Design review of the part built by this model. Coordinates are the model's own, in mm. Face numbers are marked on the shaded views. Give positions to 0.01 mm unless a question says otherwise; leave off trailing zeros. Write each loop counter-clockwise with the first axis right and the second up, starting at its lowest first coordinate (ties: lowest second). Pieces come first, ordered by that corner, then holes. Notation, with made-up numbers: (65, -30) -> (114, -30) arc R30 cw to (114, 0) -> close; hole circle Ø3 at (46, -4). An arc over 180 degrees is marked (long way). Answer as a JSON object with one key per item and string values.
Autodesk Fusion 360 part; units mm, degrees
sketch "Sketch1" plane through (0, 0, 0) normal (0, 0, 1) x (1, 0, 0)
  line L0 (10, -60) -> (-10, -60)
  line L1 (-10, -60) -> (-10, 60)
  line L2 (-10, 60) -> (10, 60)
  line L3 (10, 60) -> (10, -60)
  line L4 (10, -60) -> (-10, 60) construction
  line L5 (-10, -60) -> (10, 60) construction
  dimension "d1" = 20
  dimension "d2" = 120
extrude "Extrude1" add sketch "Sketch1" along normal blind 12
sketch "Sketch2" plane through (0, 0, 12) normal (0, 0, 1) x (-1, 0, 0)
  line L0 (-10, -60) -> (10, -60)
  line L1 (10, -60) -> (10, 60)
  line L2 (10, 60) -> (-10, 60)
  line L3 (-10, 60) -> (-10, -60)
  circle A0 centre (0, -50) radius 2
  circle A1 centre (0, 50) radius 2
extrude "Extrude2" cut sketch "Sketch2" against normal blind 12 contours A0
sketch "Sketch3" plane through (0, 0, 12) normal (0, 0, 1) x (-1, 0, 0)
  circle A0 centre (0, -50) radius 2
  line L0 (-10, -60) -> (10, -60)
  line L1 (10, -60) -> (10, 60)
  line L2 (10, 60) -> (-10, 60)
  line L3 (-10, 60) -> (-10, -60)
  circle A1 centre (0, 50) radius 2
  dimension "d10" = 4
extrude "Extrude3" cut sketch "Sketch3" against normal blind 12 contours A1
sketch "Sketch4" plane through (0, 0, 12) normal (0, 0, 1) x (-1, 0, 0)
  circle A0 centre (0, 50) radius 2
  circle A1 centre (0, -50) radius 2
  line L0 (-10, -60) -> (10, -60)
  line L1 (10, -60) -> (10, 60)
  line L2 (10, 60) -> (-10, 60)
  line L3 (-10, 60) -> (-10, -60)
  circle A2 centre (0, -34) radius 2
  circle A3 centre (0, -18) radius 2
  circle A4 centre (0, -2) radius 2
  circle A5 centre (0, 14) radius 2
  circle A6 centre (0, 30) radius 2
  point P0 (0, -34)
  point P1 (0, -18)
  point P2 (0, -2)
  point P3 (0, 14)
  point P4 (0, 30)
  point P5 (0, -18)
  point P6 (0, -2)
  point P7 (0, 14)
  point P8 (0, 30)
  point P9 (0, 46)
  dimension "d15" = 0
  dimension "d16" = 80
  dimension "d19" = 0
  dimension "d20" = 80
extrude "Extrude4" cut sketch "Sketch4" against normal blind 12 contours A2 | A3 | A4 | A5 | A6
sketch "Sketch5" plane through (0, 0, 12) normal (0, 0, 1) x (-1, 0, 0)
  line L0 (-10, -60) -> (10, -60)
  line L1 (10, -60) -> (10, 60)
  line L2 (10, 60) -> (-10, 60)
  line L3 (-10, 60) -> (-10, -60)
  circle A0 centre (0, -50) radius 2
  circle A1 centre (0, 50) radius 2
  circle A2 centre (0, 30) radius 2
  circle A3 centre (0, -34) radius 2
  circle A4 centre (0, 14) radius 2
  circle A5 centre (0, -18) radius 2
  circle A6 centre (0, -2) radius 2
sketch "Sketch6" plane through (0, 0, 12) normal (0, 0, 1) x (1, 0, 0)
  circle A0 centre (0, 50) radius 1.5
  circle A1 centre (0, 18) radius 2.25
  circle A2 centre (0, 2) radius 2.5
  circle A3 centre (0, -14) radius 3
  circle A4 centre (0, -30) radius 4
  circle A5 centre (0, -50) radius 5
  dimension "d26" = 3
  dimension "d27" = 4.5
  dimension "d28" = 5
  dimension "d29" = 6
  dimension "d30" = 8
  dimension "d31" = 10
extrude "Extrude5" add sketch "Sketch5" against normal blind 12 contours A0
extrude "Extrude6" add sketch "Sketch6" along normal blind 12 contours A0
extrude "Extrude7" cut 1 faces at (-0.1827, 50.4654, 24) along direction (0, 0, -1) blind 12
sketch "Sketch7" plane through (0, 0, 12) normal (0, 0, 1) x (-1, 0, 0)
  line L0 (-10, -60) -> (10, -60)
  line L1 (10, -60) -> (10, 60)
  line L2 (10, 60) -> (-10, 60)
  line L3 (-10, 60) -> (-10, -60)
  circle A0 centre (0, 50) radius 2
  circle A1 centre (0, 30) radius 2
  circle A2 centre (0, -34) radius 2
  circle A3 centre (0, 14) radius 2
  circle A4 centre (0, -18) radius 2
  circle A5 centre (0, -2) radius 2
  circle A6 centre (0, -50) radius 1.5
  dimension "d38" = 3
extrude "Extrude8" cut sketch "Sketch7" against normal blind 12 contours A6
sketch "Sketch8" plane through (0, 0, 12) normal (0, 0, 1) x (-1, 0, 0)
  circle A0 centre (0, -50) radius 1.5
  line L0 (-10, -60) -> (10, -60)
  line L1 (10, -60) -> (10, 60)
  line L2 (10, 60) -> (-10, 60)
  line L3 (-10, 60) -> (-10, -60)
  circle A1 centre (0, 50) radius 2
  circle A2 centre (0, 30) radius 2
  circle A3 centre (0, -34) radius 2
  circle A4 centre (0, 14) radius 2
  circle A5 centre (0, -18) radius 2
  circle A6 centre (0, -2) radius 2
  circle A7 centre (0, -18) radius 2.25
  circle A8 centre (0, -2) radius 2.5
  circle A9 centre (0, 14) radius 3
  circle A10 centre (0, 30) radius 4
  circle A11 centre (0, 50) radius 5
  dimension "d41" = 4.5
  dimension "d42" = 5
  dimension "d43" = 6
  dimension "d44" = 8
  dimension "d45" = 10
extrude "Extrude9" cut sketch "Sketch8" against normal blind 12 contours A11
sketch "Sketch9" plane through (0, 0, 12) normal (0, 0, 1) x (-1, 0, 0)
  circle A0 centre (0, -2) radius 2
  circle A1 centre (0, -18) radius 2
  circle A2 centre (0, 14) radius 2
  circle A3 centre (0, -34) radius 2
  circle A4 centre (0, 30) radius 2
  line L0 (-10, -60) -> (10, -60)
  line L1 (10, -60) -> (10, 60)
  line L2 (10, 60) -> (-10, 60)
  line L3 (-10, 60) -> (-10, -60)
  circle A5 centre (0, -50) radius 1.5
  circle A6 centre (0, 50) radius 5
  circle A7 centre (0, 30) radius 4
  dimension "d48" = 8
extrude "Extrude10" cut sketch "Sketch9" against normal blind 12 contours A7
sketch "Sketch10" plane through (0, 0, 12) normal (0, 0, 1) x (-1, 0, 0)
  circle A0 centre (0, 50) radius 5
  circle A1 centre (0, -50) radius 1.5
  line L0 (-10, -60) -> (10, -60)
  line L1 (10, -60) -> (10, 60)
  line L2 (10, 60) -> (-10, 60)
  line L3 (-10, 60) -> (-10, -60)
  circle A2 centre (0, -34) radius 2
  circle A3 centre (0, 14) radius 2
  circle A4 centre (0, -18) radius 2
  circle A5 centre (0, -2) radius 2
  circle A6 centre (0, 30) radius 4
  circle A7 centre (0, 14) radius 3
  dimension "d51" = 6
extrude "Extrude11" cut sketch "Sketch10" against normal blind 12 contours A7
sketch "Sketch11" plane through (0, 0, 12) normal (0, 0, 1) x (-1, 0, 0)
  circle A0 centre (0, 30) radius 4
  circle A1 centre (0, -2) radius 2
  circle A2 centre (0, -18) radius 2
  circle A3 centre (0, -34) radius 2
  line L0 (-10, -60) -> (10, -60)
  line L1 (10, -60) -> (10, 60)
  line L2 (10, 60) -> (-10, 60)
  line L3 (-10, 60) -> (-10, -60)
  circle A4 centre (0, -50) radius 1.5
  circle A5 centre (0, 50) radius 5
  circle A6 centre (0, 14) radius 3
  circle A7 centre (0, -2) radius 2.5
  dimension "d54" = 5
extrude "Extrude12" cut sketch "Sketch11" against normal blind 12 contours A7
sketch "Sketch12" plane through (0, 0, 12) normal (0, 0, 1) x (-1, 0, 0)
  circle A0 centre (0, 14) radius 3
  circle A1 centre (0, 50) radius 5
  circle A2 centre (0, -50) radius 1.5
  line L0 (-10, -60) -> (10, -60)
  line L1 (10, -60) -> (10, 60)
  line L2 (10, 60) -> (-10, 60)
  line L3 (-10, 60) -> (-10, -60)
  circle A3 centre (0, -34) radius 2
  circle A4 centre (0, -18) radius 2
  circle A5 centre (0, 30) radius 4
  circle A6 centre (0, -2) radius 2.5
  circle A7 centre (0, -18) radius 2.25
  dimension "d57" = 4.5
extrude "Extrude13" cut sketch "Sketch12" against normal blind 12 contours A7
fillet "Fillet1" radius 2 4 edges at (-10, -60, 6) (-10, 60, 6) (10, 60, 6) (10, -60, 6)
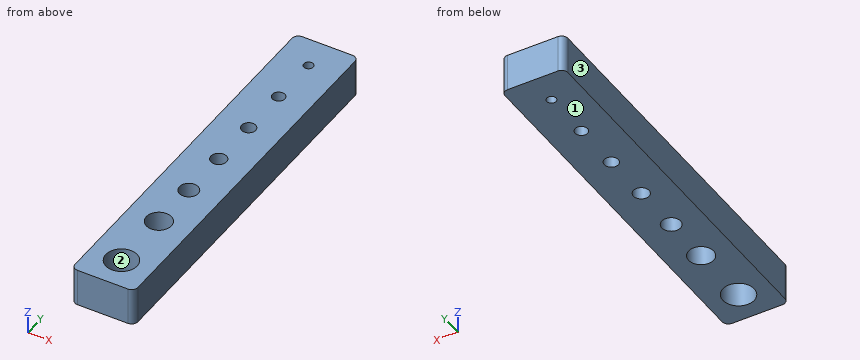
(1) We need section D-D, the plane y = 50. State the section outline as (x, z) points, then the cut area to 3 significant figures.
Here are the results:
{"outline": "(-10, 0) -> (-1.5, 0) -> (-1.5, 12) -> (-10, 12) -> close; (1.5, 0) -> (10, 0) -> (10, 12) -> (1.5, 12) -> close", "area": "204 mm²"}
(2) Clearance check with a flat-ended pin moving along its axis: pin 1 (3 mm diameter, centred on x = -6.5, y = -43, fed in from -Z). State where the tip first meets the part, or that it passes through.
Here are the results:
{"pin 1": "stops at z = 0"}
(3) For line 1 along X through (y, z) = (18, 3.75); line 2 along X through (y, z) = (34, 8.5); line 3 along Y through (x, z) = (3.5, 1.5), list the stretches that pass through material, from the lowest coordinate up.
Here are the results:
{"line 1": "x = -10 to -2.25, 2.25 to 10", "line 2": "x = -10 to -2, 2 to 10", "line 3": "y = -60 to -53.57, -46.43 to -31.94, -28.06 to 60"}
(4) We need section A-A, the plane y = 2. State the section outline as (x, z) points.
Here are the results:
{"outline": "(-10, 0) -> (-2.5, 0) -> (-2.5, 12) -> (-10, 12) -> close; (2.5, 0) -> (10, 0) -> (10, 12) -> (2.5, 12) -> close"}
(5) We need section C-C, the plane z = 9.25. State the section outline as (x, y) points.
Here are the results:
{"outline": "(-10, -58) arc R2 ccw to (-8, -60) -> (8, -60) arc R2 ccw to (10, -58) -> (10, 58) arc R2 ccw to (8, 60) -> (-8, 60) arc R2 ccw to (-10, 58) -> close; hole circle Ø10 at (0, -50); hole circle Ø8 at (0, -30); hole circle Ø6 at (0, -14); hole circle Ø5 at (0, 2); hole circle Ø4.5 at (0, 18); hole circle Ø4 at (0, 34); hole circle Ø3 at (0, 50)"}
(6) We need section B-B, the plane x = 0. Give the number of separate pieces and of enclosed holes in the cut face, then the cut area to 3 significant figures.
Here are the results:
{"separate pieces": "8", "enclosed holes": "0", "area": "954 mm²"}
(7) The part is to be moulded in two halves that separate along X. For the marked faces 1, 2 and 3, say which applies: +X half, -X half, draft (parallel to the pull), parting line (faces both ways), or undercut.
Here are the results:
{"face 1": "draft", "face 2": "undercut", "face 3": "-X half"}
